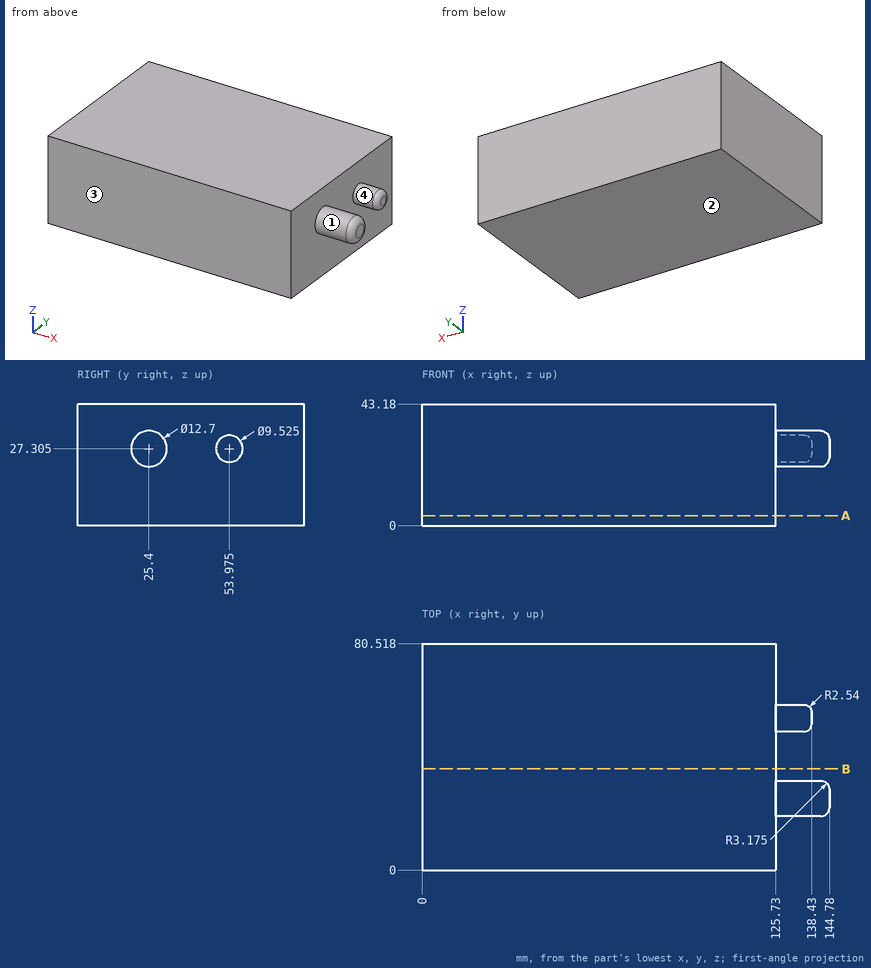
For this review, use the dimensioned drawing (mm, ordinates from the lowest corner) and the shaded views. Coordinates: 2 decimals unless noted, no trailing zeros. Loops run counter-clockwise (first coordinate to the right, second up) from the corner with the lowest first, then second, coordinate; pieces in that order, holes last. Notation, with made-up numbers: (19.25, 53) - (71.25, 53) arc R18 ccw to (71.25, 74) - close; hole circle Ø8 at (-19.75, 45). An arc over 180 degrees is marked (long way). Use one line per item in the form item = value. Start each with the question number.
1) Take a section at A-A (z = 3.5). State the section outline as (x, y) points, plus the area to 3 significant figures.
2) For pin 1 (1 mm diameter, centred on y = 29, z = 12, fed in from -X); pin 2 (21.5 mm diameter, centred on y = 41, z = 21, fed in from +X); pin 3 (1.3 mm diameter, centred on y = 54, z = 26.5, fed in from +X); pin 4 (1 mm diameter, centred on y = 45, z = 11.5, fed in from +X), all flat-tipped, find the tip position at first contact; note any pin that passes through.
3) Draft analysis for pull direction Y (two halves, no side actions). For the marked faces 1, 2, 3 and 4, state which applies: released by +Y, released by -Y, zero draft, split by the parting line, or undercut.
4) Take a section at B-B (y = 36). State the section outline as (x, z) points, plus the area to 3 significant figures.
5) To check wall thickness, follow probe 1 along X at (y, z) = (69, 33.5); probe 2 along Z at (x, y) = (135, 30.5); probe 3 along X at (y, z) = (51, 26). State the ranges of each line that lie inside material, in increasing order. Write a range as from..to.
From the geometry:
q1.outline = (0, 0) - (125.73, 0) - (125.73, 80.52) - (0, 80.52) - close
q1.area = 10,100 mm2
q2.pin_1 = 0
q2.pin_2 = 142.9
q2.pin_3 = 138.43
q2.pin_4 = 125.73
q3.face_1 = undercut
q3.face_2 = zero draft
q3.face_3 = released by -Y
q3.face_4 = undercut
q4.outline = (0, 0) - (125.73, 0) - (125.73, 43.18) - (0, 43.18) - close
q4.area = 5,430 mm2
q5.probe_1 = 0..125.73
q5.probe_2 = 23.52..31.09
q5.probe_3 = 0..138.21
